from build123d import *

# Parameters (mm, degrees)
SKETCH6_R                 = 29
SKETCH6_R_2               = 20
INNER_RING_DEPTH          = 15
MOTOR_CONNECTOR_CUT_DEPTH = 15
CUT_EXTRUDE1_DEPTH        = 16
CUT_EXTRUDE1_DEPTH_BACK   = 27
SKETCH10_R                = 3.15
CUT_EXTRUDE2_DEPTH        = 55
CUT_EXTRUDE2_DEPTH_BACK   = 70


with BuildPart() as part:
    # Sketch6 → Inner Ring (new body)
    with BuildSketch(Plane.XY):
        Circle(SKETCH6_R)
        Circle(SKETCH6_R_2, mode=Mode.SUBTRACT)
    extrude(amount=-INNER_RING_DEPTH)

    # Sketch7 → Motor Connector Cut (add)
    with BuildSketch(Plane.XY):
        with BuildLine():
            ThreePointArc((20, 0), (19.840593925, 2.52008585), (19.364916731, 5))
            Line((19.364916731, 5), (9.999996731, 5))
            Line((9.999996731, 5), (9.999996731, -5))
            Line((9.999996731, -5), (19.364916731, -5))
            ThreePointArc((19.364916731, -5), (19.840593925, -2.52008585), (20, 0))
        make_face()
        with BuildLine():
            ThreePointArc((5, 19.364916731), (0, 20), (-5, 19.364916731))
            Line((-5, 19.364916731), (-5, 9.999996731))
            Line((-5, 9.999996731), (5, 9.999996731))
            Line((5, 9.999996731), (5, 19.364916731))
        make_face()
        with BuildLine():
            Line((-9.999996731, -5), (-9.999996731, 5))
            Line((-9.999996731, 5), (-19.364916731, 5))
            ThreePointArc((-19.364916731, 5), (-20, 0), (-19.364916731, -5))
            Line((-19.364916731, -5), (-9.999996731, -5))
        make_face()
        with BuildLine():
            Line((-5, -9.999996731), (-5, -19.364916731))
            ThreePointArc((-5, -19.364916731), (0, -20), (5, -19.364916731))
            Line((5, -19.364916731), (5, -9.999996731))
            Line((5, -9.999996731), (-5, -9.999996731))
        make_face()
    extrude(amount=-MOTOR_CONNECTOR_CUT_DEPTH)

    # Sketch9 → Cut-Extrude1 (cut, two sides)
    with BuildSketch(Plane(origin=(0, 0, -15), x_dir=(-1, 0, 0), z_dir=(0, 0, -1))) as cut_extrude1_sk:
        with BuildLine():
            Line((14.5, 25.11473671), (29, 0))
            ThreePointArc((29, 0), (25.11473671, 14.5), (14.5, 25.11473671))
        make_face()
        with BuildLine():
            Line((-29, 0), (-14.5, 25.11473671))
            ThreePointArc((-14.5, 25.11473671), (-25.11473671, 14.5), (-29, 0))
        make_face()
        with BuildLine():
            ThreePointArc((-29, 0), (-25.11473671, -14.5), (-14.5, -25.11473671))
            Line((-14.5, -25.11473671), (-29, 0))
        make_face()
        with BuildLine():
            ThreePointArc((14.5, -25.11473671), (25.11473671, -14.5), (29, 0))
            Line((29, 0), (14.5, -25.11473671))
        make_face()
    extrude(amount=CUT_EXTRUDE1_DEPTH, mode=Mode.SUBTRACT)
    extrude(cut_extrude1_sk.sketch, amount=-CUT_EXTRUDE1_DEPTH_BACK, mode=Mode.SUBTRACT)

    # Sketch10 → Cut-Extrude2 (cut, two sides)
    with BuildSketch(Plane(origin=(0, 0, -15), x_dir=(-1, 0, 0), z_dir=(0, 0, -1))) as cut_extrude2_sk:
        with Locations((-17.75, 0)):
            Circle(SKETCH10_R)
        with Locations((0, 17.75)):
            Circle(SKETCH10_R)
        with Locations((17.75, 0)):
            Circle(SKETCH10_R)
        with Locations((0, -17.75)):
            Circle(SKETCH10_R)
    extrude(amount=CUT_EXTRUDE2_DEPTH, mode=Mode.SUBTRACT)
    extrude(cut_extrude2_sk.sketch, amount=-CUT_EXTRUDE2_DEPTH_BACK, mode=Mode.SUBTRACT)


solid = part.part
Source: CAD feature listing. Evaluate the final solid. Frame: model axes, mm. A direction names the side the tool comes from. Round coordinates to 2 decimals unless told otherwise and drop trailing zeros. Loops run counter-clockwise (first coordinate to the right, second up) from the corner with the lowest first, then second, coordinate; pieces in that order, holes last. Notation, with made-up numbers: (-38.5, 8.25) -> (-14.5, 8.25) arc R29 ccw to (-14.5, 41.25) -> close; hole circle Ø7 at (56, 85.25). An arc over 180 degrees is marked (long way). Answer as a JSON object with one key per item and string values. Group by question number.
Q1. Contact query for flat-ended pins moving along their axis: P1, Ø8, axis at x = 0.5, z = -6.5, coming from the -Y side; P2, Ø10, axis at x = 22.5, y = -19.5, coming from the -Z side; P3, Ø5, axis at y = 0, z = -9, coming from the -X side; P4, Ø5, axis at x = 0.5, z = -7, coming from the +Y side. Output: stop coordinate, or through.
Q2. Section query D-D (y = 12). Output: boundary loops of the cut face in (x, z), plus the area to 3 significant figures.
Q3. Mould query, pull axis X, two halves, no side actions, for faces 1 (the flat face through (21.851, 12.382, -7.605)), 2 (the cylindrical face through (0, -29, -7)), 3 (the flat face through (4, 11, -15)), 4 (the cylindrical face through (-14.6, 0.1, -7.6)). Classes: pulls with the +X half, pulls with the -X half, needs draft (parallel to the pull), parting line crosses it, or undercut.
Q4. Ray query, line 1 (Y direction, x = 0, z = -8.25); line 2 (Y direction, x = -17.75, z = -4.25); line 3 (X direction, y = 15, z = -1.25). Return the intervals inside material, ascending. Write a range as from..to.
Q5. Section query B-B (y = -7.5). Output: boundary loops of the cut face in (x, z).
Q6. Section query A-A (x = 0). Output: boundary loops of the cut face in (y, z).
Q7. Section query C-C (z = -9.75). Output: boundary loops of the cut face in (x, y), plus the area to 3 significant figures.
Q8. Access query for faces 5 (the flat face through (15, 5, -7)), 6 (the cylindrical face through (0, 29, -7)). Directions: +Z, -Z, +X, -X, +Y, -Y. A direction counts if a zero-diameter tool reaches every point of the face in a straight line with its end or side. Return the directions, or none.
Completed:
{
 "1": {"P1": "y = -29", "P2": "z = -15", "P3": "x = -29", "P4": "y = 29"},
 "2": {"outline": "(-22.07, -15) -> (-16, -15) -> (-16, 0) -> (-22.07, 0) -> close; (-5, -15) -> (5, -15) -> (5, 0) -> (-5, 0) -> close; (16, -15) -> (22.07, -15) -> (22.07, 0) -> (16, 0) -> close", "area": "332 mm²"},
 "3": {"face 1": "pulls with the +X half", "face 2": "parting line crosses it", "face 3": "needs draft", "face 4": "undercut"},
 "4": {"line 1": "-29..-20.9, -14.6..-10, 10..14.6, 20.9..29", "line 2": "-19.49..-9.22, -5..-3.15, 3.15..5, 9.22..19.49", "line 3": "-20.34..-13.23, -5..-1.54, 1.54..5, 13.23..20.34"},
 "5": {"outline": "(-24.67, -15) -> (-18.54, -15) -> (-18.54, 0) -> (-24.67, 0) -> close; (18.54, -15) -> (24.67, -15) -> (24.67, 0) -> (18.54, 0) -> close"},
 "6": {"outline": "(-29, -15) -> (-20.9, -15) -> (-20.9, 0) -> (-29, 0) -> close; (-14.6, -15) -> (-10, -15) -> (-10, 0) -> (-14.6, 0) -> close; (10, -15) -> (14.6, -15) -> (14.6, 0) -> (10, 0) -> close; (20.9, -15) -> (29, -15) -> (29, 0) -> (20.9, 0) -> close"},
 "7": {"outline": "(-29, 0) -> (-14.5, -25.11) arc R29 ccw to (14.5, -25.11) -> (29, 0) -> (14.5, 25.11) arc R29 ccw to (-14.5, 25.11) -> close; hole circle Ø6.3 at (-17.75, 0); hole (-19.36, -5) arc R20 ccw to (-5, -19.36) -> (-5, -10) -> (5, -10) -> (5, -19.36) arc R20 ccw to (19.36, -5) -> (10, -5) -> (10, 5) -> (19.36, 5) arc R20 ccw to (5, 19.36) -> (5, 10) -> (-5, 10) -> (-5, 19.36) arc R20 ccw to (-19.36, 5) -> (-10, 5) -> (-10, -5) -> close; hole circle Ø6.3 at (0, -17.75); hole circle Ø6.3 at (0, 17.75); hole circle Ø6.3 at (17.75, 0)", "area": "1,350 mm²"},
 "8": {"face 5": "+Z, -Z", "face 6": "+Z, -Z, +Y"}
}
